```python
from build123d import *

# Parameters (mm, degrees)
F1_R     = 31.75
F2_DEPTH = 6.35
F0_R     = 31.75
F3_DEPTH = 6.35
F4_DEPTH = 6.35


with BuildPart() as f2:
    # F1 (on Right) → F2 (new body)
    with BuildSketch(Plane.YZ):
        Circle(F1_R)
        Polygon((-2.4019205729, -14.036842106), (-8.4443424479, -14.036842106), (-10.3600911458, -7.7397587727), (-20.0025, -7.7397587727), (-21.9182486979, -14.036842106), (-27.9606705729, -14.036842106), (-18.6250130208, 12.5174026857), (-11.7723046875, 12.5174026857), align=None, mode=Mode.SUBTRACT)
        Polygon((25.0025882936, 12.4073878214), (25.0025882936, -14.0424445271), (19.4104372652, -14.0424445271), (19.4104372652, -2.6265834216), (8.9381792835, -2.6265834216), (8.9381792835, -14.0424445271), (3.3286613264, -14.0424445271), (3.3286613264, 12.4073878214), (8.9381792835, 12.4073878214), (8.9381792835, 2.0393314117), (19.4104372652, 2.0393314117), (19.4104372652, 12.4073878214), align=None, mode=Mode.SUBTRACT)
    extrude(amount=F2_DEPTH)

    # F0 (on Right) → F3 (join)
    with BuildSketch(Plane.YZ):
        Circle(F0_R)
    extrude(amount=-F3_DEPTH)

    # F1 (on Right) → F4 (join)
    with BuildSketch(Plane.YZ):
        with BuildLine():
            Line((-18.5902864583, -3.0400973143), (-11.7028515625, -3.0400973143))
            add(Edge.make_bspline(
                [(-11.7028515625, -3.0400973143), (-14.3594335937, 5.5142125815), (-14.6951236979, 6.6370381023)],
                knots=[0, 0, 0, 1, 1, 1], degree=2))
            add(Edge.make_bspline(
                [(-14.6951236979, 6.6370381023), (-15.0308138021, 7.7598636232), (-15.1755078125, 8.4080927898)],
                knots=[0, 0, 0, 1, 1, 1], degree=2))
            add(Edge.make_bspline(
                [(-15.1755078125, 8.4080927898), (-15.7716471354, 6.0929886232), (-18.5902864583, -3.0400973143)],
                knots=[0, 0, 0, 1, 1, 1], degree=2))
        make_face()
    extrude(amount=F4_DEPTH)

    # F6 (on offset) → F7 (revolve)
    with BuildSketch(Plane.YZ.offset(3.175)):
        with BuildLine():
            ThreePointArc((0, 33.324831301), (-1.1225320151, 30.6147992858), (1.5875, 31.737331301))
            ThreePointArc((1.5875, 31.737331301), (1.1225320151, 32.8598633161), (0, 33.324831301))
        make_face()
    revolve(axis=Axis((3.175, -10.2093983442, 34.912331301), (0, -1, 0)))


solid = f2.part
```
Design review of the part built by this model. Coordinates are the model's own, in mm. A direction names the side the tool comes from. Round coordinates to 2 decimals unless told otherwise and drop trailing zeros. Order: outer loops, then holes, each group sorted by start corner. A loop starts at its lowest first (then second) coordinate and runs counter-clockwise, first axis right, second up. Notation, with made-up numbers: (-37, -25.5) - (2, -25.5) arc R10 cw to (2, -20.5) - close; hole circle Ø3 at (47, 44). An arc over 180 degrees is marked (long way). One line per question, with ' | ' between items.
Item 1: Wall thickness on line 1 (Y direction, x = 5.25, z = -5.5); line 2 (X direction, y = 10.5, z = 29); line 3 (Z direction, x = 2, y = 22): over which ranges is each line inside the solid? List them lowest first. Write a range as [from, to].
Checks:
line 1: [-31.27, -24.96], [-5.41, 3.33], [8.94, 19.41], [25, 31.27] | line 2: [-6.35, 6.35] | line 3: [-22.89, -14.04], [12.41, 22.89]
Item 2: Take a section at A-A, the plane z = -4.5. Write out the cut boundary in (x, y).
Checks:
outline: (-6.35, -31.43) - (6.35, -31.43) - (6.35, -24.61) - (0, -24.61) - (0, -5.77) - (6.35, -5.77) - (6.35, 3.33) - (0, 3.33) - (0, 8.94) - (6.35, 8.94) - (6.35, 19.41) - (0, 19.41) - (0, 25) - (6.35, 25) - (6.35, 31.43) - (-6.35, 31.43) - close
Item 3: For P1, Ø3, axis at x = 3, z = 4.5, coming from the -Y side; P2, Ø6.5, axis at x = 3, y = -25, coming from the +Z side; P3, Ø1.9, axis at x = 3, y = -16, coming from the -Z side, all flat-tipped, find the tip position at first contact; note any pin that passes through.
Checks:
P1: y = -31.61 | P2: z = 23.13 | P3: z = -27.96
Item 4: Take a section at C-C, the plane x = 1. Give the number of separate pieces and of enclosed holes in the cut face, then the cut area to 3 significant figures.
Checks:
separate pieces: 2 | enclosed holes: 2 | area: 2,520 mm²
Item 5: Take a section at B-B, the plane x = -2.75. Write out the cut boundary in (y, z), then the cut area to 3 significant figures.
Checks:
outline: circle Ø63.5 at (0, 0) | area: 3,170 mm²
Item 6: Take a section at D-D, the plane z = -24. Write out the cut boundary in (x, y).
Checks:
outline: (-6.35, -20.79) - (6.35, -20.79) - (6.35, 20.79) - (-6.35, 20.79) - close
Item 7: Machinability: for faces 1 (the face through (6.35, -15, 1)), 2 (the face through (3, 25.003, -1)), which of the approach directions +Z, -Z, +X, -X, +Y, -Y give a long, thin tool a straight path to every point of the face, cutting with its end or side? Answer none if there is none.
Checks:
face 1: +Z, -Z, +X, +Y, -Y | face 2: +X
Item 8: Draft analysis for pull direction Z (two halves, no side actions). For faces 3 (the face through (3, 8.938, 7)), 4 (the face through (6.35, 0, 0)), 5 (the face through (3, 22, -14.042)), state which applies: +Z half, -Z half, draft (parallel to the pull), parting line (faces both ways), or undercut.
Checks:
face 3: undercut | face 4: draft | face 5: undercut
